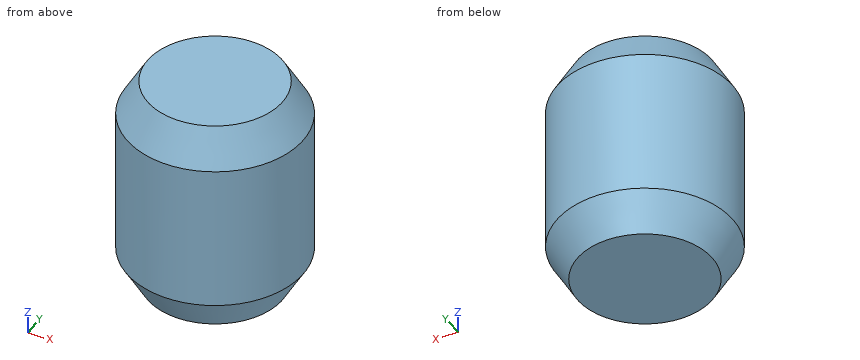
```python
from build123d import *

# Parameters (mm, degrees)
F0_R       = 30
F0_R_2     = 23
F1_DEPTH   = 74
F2_SIZE2   = 12
F2_SIZE    = 7
F2_2_SIZE2 = 12
F2_2_SIZE  = 7


with BuildPart() as f1:
    # F0 (on Top) → F1 (new body)
    with BuildSketch(Plane.XY):
        Circle(F0_R)
        Circle(F0_R_2, mode=Mode.SUBTRACT)
        Circle(F0_R_2)
    extrude(amount=F1_DEPTH)

    # F2
    f2_edges = [f1.edges().sort_by_distance(p)[0] for p in [
        (-30, 0, 74),
    ]]
    f2_side = f1.faces().sort_by_distance((0, 0, 74))[0]
    chamfer(f2_edges, length=F2_SIZE, length2=F2_SIZE2, reference=f2_side)

    # F2#2
    f2_2_edges = [f1.edges().sort_by_distance(p)[0] for p in [
        (-30, 0, 0),
    ]]
    f2_2_side = f1.faces().sort_by_distance((0, 0, 0))[0]
    chamfer(f2_2_edges, length=F2_2_SIZE, length2=F2_2_SIZE2, reference=f2_2_side)


solid = f1.part
```
The model under review builds one solid part; all positions refer to its coordinate system, in mm. Coordinates: 2 decimals unless noted, no trailing zeros. Write each loop counter-clockwise with the first axis right and the second up, starting at its lowest first coordinate (ties: lowest second). Pieces come first, ordered by that corner, then holes. Notation, with made-up numbers: (-21.75, 6.25) -> (-4.75, 6.25) arc R30 cw to (-4.75, 34.25) -> close; hole circle Ø3 at (-17, 44). An arc over 180 degrees is marked (long way). One line per item, written item: value. Start each with the question number.
Q1. Clearance check with flat-ended pins moving along their axes: P1, Ø6, axis at x = -10, z = 20.5, coming from the +Y side; P2, Ø6, axis at x = 3.5, y = -5, coming from the -Z side; P3, Ø3, axis at y = -9.5, z = 54, coming from the -X side; P4, Ø2, axis at x = 22.5, y = -16.5, coming from the +Z side. State where each tip first meets the part, or that it passes through.
Q2. Add section C-C, the plane z = 29. Give the boundary of the cut face in (x, y), then the cut area to 3 significant figures.
Q3. Add section A-A, the plane y = 0. Give the boundary of the cut face in (x, z), then the cut area to 3 significant figures.
Q4. To check wall thickness, follow probe 1 along Y at (x, z) = (1, 25); probe 2 along Y at (x, z) = (-3, 19); probe 3 along X at (y, z) = (-7, 44). State the ranges of each line that lie inside material, in increasing order.
Response:
1. P1: y = 29.17
1. P2: z = 0
1. P3: x = -28.91
1. P4: z = 67.31
2. outline: circle Ø60 at (0, 0)
2. area: 2,830 mm²
3. outline: (-30, 12) -> (-23, 0) -> (23, 0) -> (30, 12) -> (30, 62) -> (23, 74) -> (-23, 74) -> (-30, 62) -> close
3. area: 4,270 mm²
4. probe 1: -29.98 to 29.98
4. probe 2: -29.85 to 29.85
4. probe 3: -29.17 to 29.17
